```python
from build123d import *

# Parameters (mm, degrees)
SKETCH_1_W          = 20
SKETCH_1_H          = 60
SKETCH_1_R          = 4.5
EXTRUDE_1_DEPTH     = 3
EXTRUDE_2_DEPTH     = 3
EXTRUDE_START       = -3
EXTRUDE_3_DEPTH     = 3
FILLET_2_R          = 10
FILLET_3_R          = 20
FILLET_4_R          = 3
SKETCH_5_W          = 8
SKETCH_5_H          = 3
CUT_EXTRUDE_1_DEPTH = 319.896926922
SKETCH_7_R          = 1.5
CUT_EXTRUDE_2_DEPTH = 319.896926922
CUT_EXTRUDE_4_DEPTH = 10
EXTRUDE_4_DEPTH     = 3
FILLET_5_R          = 10
FILLET_6_R          = 10
FILLET_7_R          = 5
SKETCH_11_R         = 1.5
CUT_EXTRUDE_6_DEPTH = 319.896926922
SKETCH_12_R         = 1.5
CUT_EXTRUDE_7_DEPTH = 319.896926922


with BuildPart() as part:
    # 草图1 → 凸台-拉伸1 (new body)
    with BuildSketch(Plane.XY):
        with Locations((0, 19)):
            Rectangle(SKETCH_1_W, SKETCH_1_H)
        Circle(SKETCH_1_R, mode=Mode.SUBTRACT)
        with Locations((0, 38)):
            Circle(SKETCH_1_R, mode=Mode.SUBTRACT)
    extrude(amount=EXTRUDE_1_DEPTH)

    # 草图3 → 凸台-拉伸2 (add)
    with BuildSketch(Plane.XY.offset(3)):
        with BuildLine():
            Line((-10, 100.977093724), (-10, 79.00084746))
            ThreePointArc((-10, 79.00084746), (0.177205293, 83.704863402), (10, 89.110044035))
            ThreePointArc((10, 89.110044035), (67.140217047, 147.506329367), (88, 226.5))
            ThreePointArc((88, 226.5), (82.919333848, 266.5), (68, 303.959666924))
            Line((68, 303.959666924), (68, 226.5))
            ThreePointArc((68, 226.5), (46.91173197, 152.608187192), (-10, 100.977093724))
        make_face()
        with BuildLine():
            Line((-10, 79.00084746), (-10, 49))
            Line((-10, 49), (10, 49))
            Line((10, 49), (10, 89.110044035))
            ThreePointArc((10, 89.110044035), (0.177205293, 83.704863402), (-10, 79.00084746))
        make_face()
        with BuildLine():
            Line((68, 306.5), (68, 303.959666924))
            ThreePointArc((68, 303.959666924), (82.919333848, 266.5), (88, 226.5))
            Line((88, 226.5), (88, 306.5))
            Line((88, 306.5), (68, 306.5))
        make_face()
    extrude(amount=-EXTRUDE_2_DEPTH)

    # 草图4 → 凸台-拉伸3 (add)
    with BuildSketch(Plane(origin=(0, 0, 0), x_dir=(-1, 0, 0), z_dir=(0, 0, -1)).offset(EXTRUDE_START)):
        with BuildLine():
            Line((-40, -11), (-10, -11))
            Line((-10, -11), (-10, -1))
            Line((-10, -1), (-30, -1))
            Line((-30, -1), (-59.811855282, 135.804714527))
            ThreePointArc((-59.811855282, 135.804714527), (-74.827433124, 162.925595698), (-84.331190721, 192.433024677))
            Line((-84.331190721, 192.433024677), (-40, -11))
        make_face()
    extrude(amount=EXTRUDE_3_DEPTH)

    # 圆角2
    fillet_2_edges = [part.edges().sort_by_distance(p)[0] for p in [
        (88, 306.5, 1.5),
        (40, -11, 1.5),
        (-10, -11, 1.5),
    ]]
    fillet(fillet_2_edges, radius=FILLET_2_R)

    # 圆角3
    fillet_3_edges = [part.edges().sort_by_distance(p)[0] for p in [
        (-10, 100.977093724, 1.5),
    ]]
    fillet(fillet_3_edges, radius=FILLET_3_R)

    # 圆角4
    fillet_4_edges = [part.edges().sort_by_distance(p)[0] for p in [
        (68, 306.5, 1.5),
    ]]
    fillet(fillet_4_edges, radius=FILLET_4_R)

    # 草图5 → 切除-拉伸1 (cut, through all)
    with BuildSketch(Plane.XY.offset(3)):
        Polygon((46.77842194, 43.588901874), (43.847212114, 44.227657662), (42.143863348, 36.411098126), (45.075073174, 35.772342338), align=None)
        Polygon((70.199467474, 151.066595495), (68.496118708, 143.250035959), (65.564908882, 143.888791747), (67.268257648, 151.705351283), align=None)
        with Locations((28, 115)):
            Rectangle(SKETCH_5_W, SKETCH_5_H)
        Polygon((79.767766953, 280.389087297), (74.110912703, 274.732233047), (76.232233047, 272.610912703), (81.889087297, 278.267766953), align=None)
        Polygon((79.767766953, 230.389087297), (81.889087297, 228.267766953), (76.232233047, 222.610912703), (74.110912703, 224.732233047), align=None)
    extrude(amount=-CUT_EXTRUDE_1_DEPTH, mode=Mode.SUBTRACT)

    # 草图7 → 切除-拉伸2 (cut, through all)
    with BuildSketch(Plane(origin=(0, 0, 0), x_dir=(-1, 0, 0), z_dir=(0, 0, -1))):
        with Locations((-72.125207072, 166.801384551)):
            Circle(SKETCH_7_R)
        with Locations((-75.700287711, 195.105334687)):
            Circle(SKETCH_7_R)
        with Locations(Location((-54.63925576, 144.259505713, 0), (0, 0, 180))):
            Circle(SKETCH_7_R)
    extrude(amount=-CUT_EXTRUDE_2_DEPTH, mode=Mode.SUBTRACT)

    # 草图8 → 切除-拉伸4 (cut)
    with BuildSketch(Plane.XY.offset(3)):
        Polygon((37.268809589, 32.356106534), (48.895829905, 29.822399649), (39.17112789, -58.646231881), (10, -11), (10, -1), align=None)
    extrude(amount=-CUT_EXTRUDE_4_DEPTH, mode=Mode.SUBTRACT)

    # 草图9 → 凸台-拉伸4 (add)
    with BuildSketch(Plane.XY.offset(3)):
        Polygon((48.895829905, 29.822399649), (10, -11), (10, -0.039068456), (10, 6.39592954), (38.020150061, 35.803960345), (37.268809589, 32.356106534), align=None)
    extrude(amount=-EXTRUDE_4_DEPTH)

    # 圆角5
    fillet_5_edges = [part.edges().sort_by_distance(p)[0] for p in [
        (10, -11, 1.5),
        (48.895829905, 29.822399649, 1.5),
    ]]
    fillet(fillet_5_edges, radius=FILLET_5_R)

    # 圆角6
    fillet_6_edges = [part.edges().sort_by_distance(p)[0] for p in [
        (10, 89.110044035, 1.5),
        (59.811855282, 135.804714527, 1.5),
    ]]
    fillet(fillet_6_edges, radius=FILLET_6_R)

    # 圆角7
    fillet_7_edges = [part.edges().sort_by_distance(p)[0] for p in [
        (10, 6.39592954, 1.5),
        (38.020150061, 35.803960345, 1.5),
    ]]
    fillet(fillet_7_edges, radius=FILLET_7_R)

    # 草图11 → 切除-拉伸6 (cut, through all)
    with BuildSketch(Plane.XY.offset(3)):
        with Locations((24, 115)):
            Circle(SKETCH_11_R)
        with Locations((32, 115)):
            Circle(SKETCH_11_R)
        with Locations((43.609468261, 36.091720232)):
            Circle(SKETCH_11_R)
        with Locations((45.312817027, 43.908279768)):
            Circle(SKETCH_11_R)
        with Locations((67.030513795, 143.569413853)):
            Circle(SKETCH_11_R)
        with Locations((68.733862561, 151.385973389)):
            Circle(SKETCH_11_R)
        with Locations((80.828427125, 229.328427125)):
            Circle(SKETCH_11_R)
        with Locations((75.171572875, 223.671572875)):
            Circle(SKETCH_11_R)
        with Locations((80.828427125, 279.328427125)):
            Circle(SKETCH_11_R)
        with Locations((75.171572875, 273.671572875)):
            Circle(SKETCH_11_R)
    extrude(amount=-CUT_EXTRUDE_6_DEPTH, mode=Mode.SUBTRACT)

    # 草图12 → 切除-拉伸7 (cut, through all)
    with BuildSketch(Plane(origin=(0, 0, 0), x_dir=(-1, 0, 0), z_dir=(0, 0, -1))):
        with Locations((-78, 291.5)):
            Circle(SKETCH_12_R)
        with Locations((-78, 266.5)):
            Circle(SKETCH_12_R)
        with Locations((-78, 241.5)):
            Circle(SKETCH_12_R)
    extrude(amount=-CUT_EXTRUDE_7_DEPTH, mode=Mode.SUBTRACT)


solid = part.part
```
Geometry: final body of the model. Coordinates: model frame, mm. A direction names the side the tool comes from. Round coordinates to 2 decimals unless told otherwise and drop trailing zeros. Loops run counter-clockwise (first coordinate to the right, second up) from the corner with the lowest first, then second, coordinate; pieces in that order, holes last. Notation, with made-up numbers: (23.5, -23.75) -> (27.5, -23.75) arc R32 ccw to (27.5, 10.25) -> close; hole circle Ø6 at (26, 57.25). An arc over 180 degrees is marked (long way). Use one line per item in the form item = value.
Item 1: Draft query along X for faces 1 (the cylindrical face through (-7.463, 98.858, 1.479)), 2 (the flat face through (27.708, 24.981, 1.521)), 3 (the flat face through (39, 137, 0)), 4 (the cylindrical face through (85.15, 303.49, 1.48)). Return one class per face: released by +X, released by -X, zero draft, split by the parting line, or undercut.
Evaluation:
face_1 = released by -X
face_2 = undercut
face_3 = zero draft
face_4 = released by +X
Item 2: Material intervals for probe 1 along Y at (x, z) = (3, 0.7); probe 2 along X at (y, z) = (252.5, 1.65); probe 3 along X at (y, z) = (114.5, 0.8), sorted ascending.
Evaluation:
probe_1 = -11 to -3.35, 3.35 to 34.65, 41.35 to 108.28
probe_2 = 68 to 88
probe_3 = 12 to 22.59, 33.41 to 67.35
Item 3: Access query for faces 5 (the flat face through (76.9, 227.52, 1.52)), 6 (the cylindrical face through (50.244, 158.262, 1.521)). Directions: +Z, -Z, +X, -X, +Y, -Y. A direction counts if a zero-diameter tool reaches every point of the face in a straight line with its end or side. Return the directions, or none.
Evaluation:
face_5 = +Z, -Z
face_6 = +Z, -Z, -X, +Y
Item 4: Contact query for flat-ended pins moving along their axis: pin 1 Ø1.8 at (x, y) = (72.13, 166.8) entering from -Z; pin 2 Ø0.9 at (x, z) = (26, 2) entering from -Y; pin 3 Ø1.5 at (x, z) = (28.5, 1.5) entering from +Y. Output: stop coordinate, or through.
Evaluation:
pin_1 = through
pin_2 = 5.32
pin_3 = 129.81
Item 5: Cut plane C-C on y = 156. Output: boundary loops of the cut face in (x, z).
Evaluation:
outline = (48.95, 0) -> (76.39, 0) -> (76.39, 3) -> (48.95, 3) -> close
Item 6: Cut plane B-B on y = 246. Output: boundary loops of the cut face in (x, z).
Evaluation:
outline = (68, 0) -> (88, 0) -> (88, 3) -> (68, 3) -> close
Item 7: Cut plane A-A on y = 53. Output: boundary loops of the cut face in (x, z).
Evaluation:
outline = (-10, 0) -> (10, 0) -> (10, 3) -> (-10, 3) -> close; (41.77, 0) -> (53.95, 0) -> (53.95, 3) -> (41.77, 3) -> close
